Study the drawing (mm; zero at the part's minimum x, y, z) and answer. Give positions to 0.01 mm unless a question says otherwise; leave off trailing zeros. Order: outer loops, then holes, each group sorted by start corner. A loop starts at its lowest first (then second) coordinate and runs counter-clockwise, first axis right, second up. Notation, with made-up numbers: (28.25, 4.25) -> (34.25, 4.25) arc R22 ccw to (34.25, 35.25) -> close; hole circle Ø2 at (51.5, 82.25). An arc over 180 degrees is marked (long way). Use a Markdown table: item, result. Add a question column.
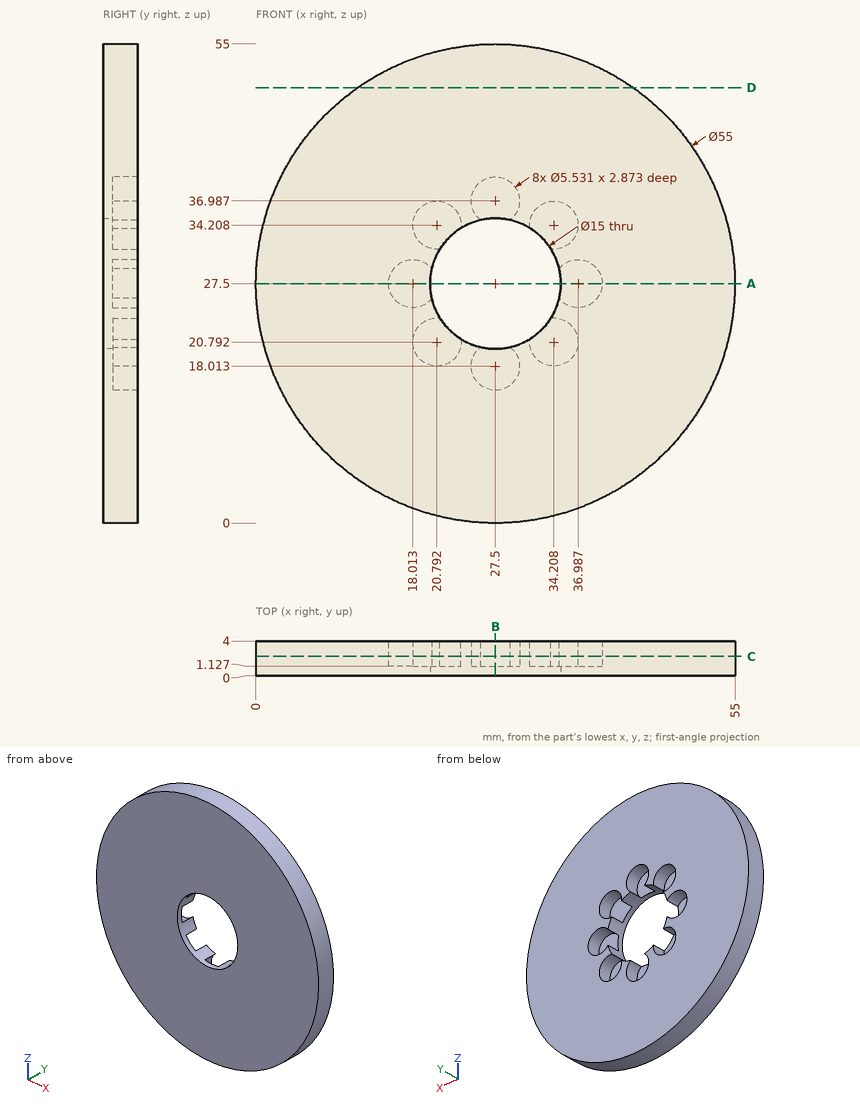
1) The part is cut by section C-C, the plane y = 2.25. Determine the outline of the cut face in (x, z) (1 decimal), then the cut area to 3 significant figures.
2) The part is cut by section D-D, the plane z = 50. Determine the outline of the cut face in (x, y).
3) The part is cut by section A-A, the plane z = 27.5. Determine the outline of the cut face in (x, y), then the cut area to 3 significant figures.
4) The part is cut by section B-B, the plane x = 27.5. Determine the outline of the cut face in (y, z).
5) Straight lines are drawn through the part: line 1 (Z direction, x = 25.5, y = 3.7) (1 decimal); line 2 (Z direction, x = 19.5, y = 2.95) (1 decimal); line 3 (Z direction, x = 33.5, y = 2.3). For each, find the intervals that lie inside material, in ascending order.
6) Flat-ended cylindrical pins translate along their axes: pin 1 (1.5 mm diameter, centred on x = 28, z = 36.5, fed in from +Y); pin 2 (1.5 mm diameter, centred on y = 1.5, z = 39.5, fed in from +X); pin 3 (1 mm diameter, centred on y = 3.5, z = 8, fed in from -X). Find the tip coordinate at first contact, or state that the pin passes through.
A:
| question | item | result |
|---|---|---|
| 1 | outline | circle Ø55 at (27.5, 27.5); hole (20.2, 25.8) arc R7.5 ccw to (21.1, 23.5) arc R2.8 ccw (long way) to (23.5, 21.1) arc R7.5 ccw to (25.8, 20.2) arc R2.8 ccw (long way) to (29.2, 20.2) arc R7.5 ccw to (31.5, 21.1) arc R2.8 ccw (long way) to (33.9, 23.5) arc R7.5 ccw to (34.8, 25.8) arc R2.8 ccw (long way) to (34.8, 29.2) arc R7.5 ccw to (33.9, 31.5) arc R2.8 ccw (long way) to (31.5, 33.9) arc R7.5 ccw to (29.2, 34.8) arc R2.8 ccw (long way) to (25.8, 34.8) arc R7.5 ccw to (23.5, 33.9) arc R2.8 ccw (long way) to (21.1, 31.5) arc R7.5 ccw to (20.2, 29.2) arc R2.8 ccw (long way) to start |
| 1 | area | 2,020 mm^2 |
| 2 | outline | (11.69, 0) -> (43.31, 0) -> (43.31, 4) -> (11.69, 4) -> close |
| 3 | outline | (0, 0) -> (20, 0) -> (20, 1.13) -> (15.25, 1.13) -> (15.25, 4) -> (0, 4) -> close; (35, 0) -> (55, 0) -> (55, 4) -> (39.75, 4) -> (39.75, 1.13) -> (35, 1.13) -> close |
| 3 | area | 133 mm^2 |
| 4 | outline | (0, 0) -> (4, 0) -> (4, 15.25) -> (1.13, 15.25) -> (1.13, 20) -> (0, 20) -> close; (0, 35) -> (1.13, 35) -> (1.13, 39.75) -> (4, 39.75) -> (4, 55) -> (0, 55) -> close |
| 5 | line 1 | 0.1 to 16.1, 19.9 to 20.3, 34.7 to 35.1, 38.9 to 54.9 |
| 5 | line 2 | 1.2 to 18.3, 23.2 to 25.2, 29.8 to 31.8, 36.7 to 53.8 |
| 5 | line 3 | 0.66 to 18.12, 36.88 to 54.34 |
| 6 | pin 1 | y = 1.13 |
| 6 | pin 2 | x = 52.59 |
| 6 | pin 3 | x = 7.62 |
